Geometry: final body of the model. Coordinates: model frame, mm. Give positions to 0.01 mm unless a question says otherwise; leave off trailing zeros. Write each loop counter-clockwise with the first axis right and the second up, starting at its lowest first coordinate (ties: lowest second). Pieces come first, ordered by that corner, then holes.
```python
from build123d import *

# Parameters (mm, degrees)
SKETCH_1_R      = 5
EXTRUDE_1_DEPTH = 4
SKETCH_2_R      = 6
EXTRUDE_2_DEPTH = 1
SKETCH_4_R      = 6
SKETCH_4_R_2    = 5
EXTRUDE_3_DEPTH = 1


with BuildPart() as part:
    # Эскиз1 → Бобышка-Вытянуть1 (new body)
    with BuildSketch(Plane(origin=(0, 0, 0), x_dir=(1, 0, 0), z_dir=(0, 1, 0))):
        with BuildLine():
            ThreePointArc((-5.5, -2.397915762), (6, 0), (-5.5, 2.397915762))
            ThreePointArc((-5.5, 2.397915762), (-17, 0), (-5.5, -2.397915762))
        make_face()
        with Locations(Location((0, 0, 0), (0, 0, 270))):
            Circle(SKETCH_1_R, mode=Mode.SUBTRACT)
        with Locations(Location((-11, 0, 0), (0, 0, 270))):
            Circle(SKETCH_1_R, mode=Mode.SUBTRACT)
    extrude(amount=EXTRUDE_1_DEPTH)

    # Эскиз2 → Бобышка-Вытянуть2 (add)
    with BuildSketch(Plane.XZ):
        Circle(SKETCH_2_R)
    extrude(amount=-EXTRUDE_2_DEPTH)

    # Эскиз4 → Бобышка-Вытянуть3 (add)
    with BuildSketch(Plane(origin=(0, 4, 0), x_dir=(1, 0, 0), z_dir=(0, 1, 0))):
        with Locations(Location((0, 0, 0), (0, 0, 156.443535691))):
            Circle(SKETCH_4_R)
        with Locations(Location((0, 0, 0), (0, 0, 90))):
            Circle(SKETCH_4_R_2, mode=Mode.SUBTRACT)
    extrude(amount=EXTRUDE_3_DEPTH)


solid = part.part
```
Item 1: Line query: L1, parallel to X at y = 2.4, z = 0; L2, parallel to X at y = 4.5, z = 0. Output: solid intervals per line, ascending.
Found:
L1: x = -17 to -16, -6 to -5, 5 to 6
L2: x = -6 to -5, 5 to 6
Item 2: Pin query (flat end, axial travel): pin 1 Ø5 at (x, z) = (0, 1.5) entering from +Y; pin 2 Ø4 at (x, z) = (1, 3.5) entering from +Y; pin 3 Ø1.5 at (y, z) = (1, 5) entering from -X. Return the tip coordinate at first contact, or that it passes through.
Found:
pin 1: stops at y = 1
pin 2: stops at y = 5
pin 3: stops at x = -15.24
Item 3: Section C-C, the plane z = -4.5. Return the cut outline in (x, y), plus the area to 3 significant figures.
Found:
outline: (-14.97, 0) - (-13.18, 0) - (-13.18, 4) - (-14.97, 4) - close; (-8.82, 0) - (-7.03, 0) - (-7.03, 4) - (-8.82, 4) - close; (-3.97, 0) - (3.97, 0) - (3.97, 5) - (2.18, 5) - (2.18, 1) - (-2.18, 1) - (-2.18, 5) - (-3.97, 5) - close
area: 36.6 mm2
Item 4: Section B-B, the plane z = -0.5. Return the cut outline in (x, y), plus the area to 3 significant figures.
Found:
outline: (-16.98, 0) - (-15.97, 0) - (-15.97, 4) - (-16.98, 4) - close; (-6.03, 0) - (5.98, 0) - (5.98, 5) - (4.97, 5) - (4.97, 1) - (-4.97, 1) - (-4.97, 5) - (-5.98, 5) - (-5.98, 4) - (-6.03, 4) - close
area: 24.2 mm2
Item 5: Pull-direction query (X, two-part tool) for faces 1 (the face through (0, 1, 0)), 2 (the face through (-3, 0, 0)); classes: +X half, -X half, draft (parallel to the pull), parting line (faces both ways), or undercut.
Found:
face 1: undercut
face 2: draft
Item 6: Section A-A, the plane x = -8.5. Return the cut outline in (y, z), plus the area to 3 significant figures.
Found:
outline: (0, -5.45) - (4, -5.45) - (4, -4.33) - (0, -4.33) - close; (0, 4.33) - (4, 4.33) - (4, 5.45) - (0, 5.45) - close
area: 8.99 mm2
Item 7: Section D-D, the plane x = 0. Return the cut outline in (y, z), plus the area to 3 significant figures.
Found:
outline: (0, -6) - (5, -6) - (5, -5) - (1, -5) - (1, 5) - (5, 5) - (5, 6) - (0, 6) - close
area: 20.0 mm2
